```python
from build123d import *

# Parameters (mm, degrees)
EXTRUDE_1_DEPTH     = 40
SKETCH_2_R          = 12
EXTRUDE_2_DEPTH     = 20
SKETCH_3_W          = 16
SKETCH_3_H          = 43
CUT_EXTRUDE_1_DEPTH = 30
SKETCH_4_R          = 5
CUT_EXTRUDE_2_DEPTH = 85.581321815
SKETCH_5_R          = 6
CUT_EXTRUDE_3_DEPTH = 16


with BuildPart() as part:
    # 草图1 → 凸台-拉伸1 (new body)
    with BuildSketch(Plane(origin=(-20, 0, 0), x_dir=(0, 0, -1), z_dir=(1, 0, 0))):
        with BuildLine():
            Line((15, 20), (-15, 20))
            Line((-15, 20), (-15, 58))
            ThreePointArc((-15, 58), (0, 73), (15, 58))
            Line((15, 58), (15, 20))
        make_face()
    extrude(amount=EXTRUDE_1_DEPTH)

    # 草图2 → 凸台-拉伸2 (add)
    with BuildSketch(Plane(origin=(0, 0, 0), x_dir=(1, 0, 0), z_dir=(0, 1, 0))):
        with Locations(Location((0, 0, 0), (0, 0, 270))):
            Circle(SKETCH_2_R)
    extrude(amount=EXTRUDE_2_DEPTH)

    # 草图3 → 切除-拉伸1 (cut)
    with BuildSketch(Plane.XY.offset(-15)):
        with Locations((0, 61.5)):
            Rectangle(SKETCH_3_W, SKETCH_3_H)
    extrude(amount=CUT_EXTRUDE_1_DEPTH, mode=Mode.SUBTRACT)

    # 草图4 → 切除-拉伸2 (cut, through all)
    with BuildSketch(Plane(origin=(-20, 0, 0), x_dir=(0, 0, -1), z_dir=(1, 0, 0))):
        with Locations(Location((0, 58, 0), (0, 0, 180))):
            Circle(SKETCH_4_R)
    extrude(amount=CUT_EXTRUDE_2_DEPTH, mode=Mode.SUBTRACT)

    # 草图5 → 切除-拉伸3 (cut)
    with BuildSketch(Plane(origin=(0, 0, 0), x_dir=(1, 0, 0), z_dir=(0, 1, 0))):
        with Locations(Location((0, 0, 0), (0, 0, 270))):
            Circle(SKETCH_5_R)
    extrude(amount=CUT_EXTRUDE_3_DEPTH, mode=Mode.SUBTRACT)


solid = part.part
```
Design review of the part built by this model. Coordinates are the model's own, in mm. A direction names the side the tool comes from. Round coordinates to 2 decimals unless told otherwise and drop trailing zeros. Write each loop counter-clockwise with the first axis right and the second up, starting at its lowest first coordinate (ties: lowest second). Pieces come first, ordered by that corner, then holes.
Item 1: The part is to be moulded in two halves that separate along Y. For faces 1 (the flat face through (-20, 47, 0)), 2 (the cylindrical face through (13.916, 53.043, -0.651)), 3 (the cylindrical face through (14, 73, 0)), say which applies: +Y half, -Y half, draft (parallel to the pull), parting line (faces both ways), or undercut.
Item 2: Clearance check with flat-ended pins moving along their axes: pin 1 Ø12 at (x, z) = (-2.5, -3.5) entering from +Y; pin 2 Ø8 at (x, z) = (0.5, 4.5) entering from +Y; pin 3 Ø1 at (x, y) = (-0.5, 10) entering from +Z. State where each tip first meets the part, or that it passes through.
Item 3: We need section A-A on z = 0. Write out the cut boundary in (x, y), and give its area (3 significant figures).
Item 4: For probe 1 along Y at (x, z) = (11.75, 0); probe 2 along Y at (x, z) = (16, 0); probe 3 along X at (y, z) = (52.5, 12.75), list the stretches that pass through material, from the lowest coordinate up.
Item 5: We need section C-C on y = 66. Write out the cut boundary in (x, z).
Item 6: We need section D-D on x = 1.5. Write out the cut boundary in (y, z), and give its area (3 significant figures).
Item 7: We need section B-B on x = 16.5. Write out the cut boundary in (y, z), and give its area (3 significant figures).
Item 8: For faces 4 (the flat face through (-14, 20, 0)), 5 (the cylindrical face through (-14, 73, 0)), 6 (the flat face through (8, 52.6, -0.2)), list the 3-axis set-ups (+Z, -Z, +X, -X, +Y, -Y) from which the entire face can be reached by the end or side of a thin tool; tool diameter is ignored.
Returned:
1. face 1: draft
1. face 2: undercut
1. face 3: +Y half
2. pin 1: stops at y = 72.96
2. pin 2: stops at y = 40
2. pin 3: stops at z = 12
3. outline: (-20, 20) - (-12, 20) - (-12, 0) - (-6, 0) - (-6, 16) - (6, 16) - (6, 0) - (12, 0) - (12, 20) - (20, 20) - (20, 53) - (8, 53) - (8, 40) - (-8, 40) - (-8, 53) - (-20, 53) - close; (-20, 63) - (-8, 63) - (-8, 73) - (-20, 73) - close; (8, 63) - (20, 63) - (20, 73) - (8, 73) - close
3. area: 1,640 mm2
4. probe 1: y = 0 to 53, 63 to 73
4. probe 2: y = 20 to 53, 63 to 73
4. probe 3: x = -20 to -8, 8 to 20
5. outline: (-20, -12.69) - (-8, -12.69) - (-8, 12.69) - (-20, 12.69) - close; (8, -12.69) - (20, -12.69) - (20, 12.69) - (8, 12.69) - close
6. outline: (0, -11.91) - (20, -11.91) - (20, -15) - (40, -15) - (40, 15) - (20, 15) - (20, 11.91) - (0, 11.91) - (0, 5.81) - (16, 5.81) - (16, -5.81) - (0, -5.81) - close
6. area: 890 mm2
7. outline: (20, -15) - (58, -15) arc R15 ccw to (58, 15) - (20, 15) - close; hole circle Ø10 at (58, 0)
7. area: 1,410 mm2
8. face 4: -Y
8. face 5: +X, -X, +Y
8. face 6: +Z, -Z, +Y
